For this review, take the finished solid that the model builds, in its own axes (mm). Face numbers are marked on the shaded views. Coordinates: 2 decimals unless noted, no trailing zeros. Loops run counter-clockwise (first coordinate to the right, second up) from the corner with the lowest first, then second, coordinate; pieces in that order, holes last.
1. Take a section at A-A, the plane z = 0. State the section outline as (x, y) points (1 decimal).
2. Take a section at D-D, the plane z = 16. State the section outline as (x, y) points (1 decimal).
3. Clearance check with flat-ended pins moving along their axes: P1, Ø1.9, axis at x = -40, z = 34, coming from the +Y side; P2, Ø3.5, axis at x = -48.006, z = 0, coming from the +Y side; P3, Ø12, axis at x = -10.5, z = 20, coming from the +Y side. State where each tip first meets the part, or that it passes through.
4. To check wall thickness, follow probe 1 along Z at (x, y) = (-13.5, -1.55); probe 2 along X at (y, z) = (-1.3, 18.5); probe 3 along Z at (x, y) = (36.5, -2.25). State the ranges of each line that lie inside material, in increasing order.
5. Take a section at C-C, the plane y = -0.95. Count the separate pieces of the cut face and the enclosed holes in it, then the cut area to 3 significant figures.
6. Mouldability with a two-part tool opening along X and no side actions: class the marked faces 1 and 2 as pulls with the +X half, pulls with the -X half, needs draft (parallel to the pull), parting line crosses it, or undercut.
7. Take a section at B-B, the plane x = 0. State the section outline as (y, z) points (1 decimal).
```python
from build123d import *

# Parameters (mm, degrees)
SKETCH1_W              = 108.712
SKETCH1_H              = 101.7524
SKETCH1_W_2            = 32.004
SKETCH1_H_2            = 38.1
BOSS_EXTRUDE1_DEPTH    = 3.175
SKETCH1_4_W            = 32.004
SKETCH1_4_H            = 38.1
CUT_EXTRUDE1_DEPTH     = 1.5875
SKETCH4_R              = 3.175
CUT_EXTRUDE2_DEPTH     = 2.5
FILLET1_R              = 7.62
F_10_32_TAPPED_HOLE1_D = 4.0386
FILLET2_R              = 3.175


with BuildPart() as part:
    # Sketch1 → Boss-Extrude1 (new body)
    with BuildSketch(Plane(origin=(0, 0, 0), x_dir=(1, 0, 0), z_dir=(0, 1, 0))):
        Rectangle(SKETCH1_W, SKETCH1_H)
        with Locations((-4.064, -9.6012)):
            Rectangle(SKETCH1_W_2, SKETCH1_H_2, mode=Mode.SUBTRACT)
        with Locations((-4.064, -9.6012)):
            Rectangle(SKETCH1_W_2, SKETCH1_H_2)
    extrude(amount=-BOSS_EXTRUDE1_DEPTH)

    # Sketch1_4 → Cut-Extrude1 (cut)
    with BuildSketch(Plane(origin=(0, 0, 0), x_dir=(1, 0, 0), z_dir=(0, 1, 0))):
        with Locations((-4.064, -9.6012)):
            Rectangle(SKETCH1_4_W, SKETCH1_4_H)
    extrude(amount=-CUT_EXTRUDE1_DEPTH, mode=Mode.SUBTRACT)

    # Sketch4 → Cut-Extrude2 (cut)
    with BuildSketch(Plane(origin=(0, 0, 0), x_dir=(1, 0, 0), z_dir=(0, 1, 0))):
        with Locations(Location((-38.481, 19.0246, 0), (0, 0, 270))):
            Circle(SKETCH4_R)
        with Locations(Location((-16.7386, 35.0012, 0), (0, 0, 270))):
            Circle(SKETCH4_R)
        with Locations(Location((38.481, 35.0012, 0), (0, 0, 270))):
            Circle(SKETCH4_R)
        with Locations(Location((38.481, -35.0012, 0), (0, 0, 270))):
            Circle(SKETCH4_R)
        with Locations(Location((-38.481, -35.0012, 0), (0, 0, 270))):
            Circle(SKETCH4_R)
    extrude(amount=-CUT_EXTRUDE2_DEPTH, mode=Mode.SUBTRACT)

    # Fillet1
    fillet1_edges = [part.edges().sort_by_distance(p)[0] for p in [
        (-54.356, -1.5875, 50.8762),
        (-54.356, -1.5875, -50.8762),
        (54.356, -1.5875, -50.8762),
        (54.356, -1.5875, 50.8762),
    ]]
    fillet(fillet1_edges, radius=FILLET1_R)

    # 10-32 Tapped Hole1 (through all)
    with Locations(Plane(origin=(0, 0, 0), x_dir=(1, 0, 0), z_dir=(0, 1, 0))):
        with Locations((-48.006, 44.5262), (48.006, 44.5262), (48.006, -44.5262), (-48.006, -44.5262), (0, -44.5262), (-48.006, 0), (48.006, 0), (0, 44.5262)):
            Hole(F_10_32_TAPPED_HOLE1_D / 2)

    # Fillet2
    fillet2_edges = [part.edges().sort_by_distance(p)[0] for p in [
        (-20.066, -0.79375, 28.6512),
        (-20.066, -0.79375, -9.4488),
        (11.938, -0.79375, -9.4488),
        (11.938, -0.79375, 28.6512),
    ]]
    fillet(fillet2_edges, radius=FILLET2_R)


solid = part.part
```
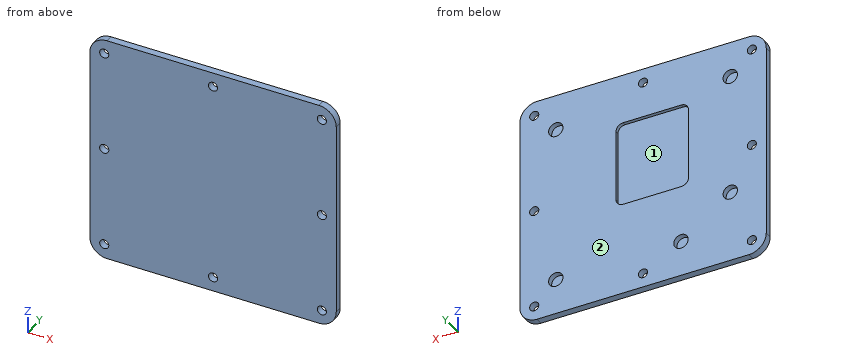
Results list:
1. outline: (-54.4, -3.2) - (-50, -3.2) - (-50, 0) - (-54.4, 0) - close; (-46, -3.2) - (46, -3.2) - (46, 0) - (11.9, 0) - (11.9, -1.6) - (-20.1, -1.6) - (-20.1, 0) - (-46, 0) - close; (50, -3.2) - (54.4, -3.2) - (54.4, 0) - (50, 0) - close
2. outline: (-54.4, -3.2) - (54.4, -3.2) - (54.4, 0) - (11.9, 0) - (11.9, -1.6) - (-20.1, -1.6) - (-20.1, 0) - (-54.4, 0) - close
3. P1: stops at y = -2.5
3. P2: passes through
3. P3: stops at y = -1.59
4. probe 1: z = -50.88 to -9.45, 28.65 to 50.88
4. probe 2: x = -54.36 to -20.07, 11.94 to 54.36
4. probe 3: z = -50.88 to -37.48, -32.52 to 32.52, 37.48 to 50.88
5. separate pieces: 1
5. enclosed holes: 14
5. area: 9,540 mm2
6. face 1: undercut
6. face 2: needs draft
7. outline: (-3.2, -50.9) - (0, -50.9) - (0, -46.5) - (-3.2, -46.5) - close; (-3.2, -42.5) - (0, -42.5) - (0, -9.4) - (-1.6, -9.4) - (-1.6, 28.7) - (0, 28.7) - (0, 42.5) - (-3.2, 42.5) - close; (-3.2, 46.5) - (0, 46.5) - (0, 50.9) - (-3.2, 50.9) - close
